Answer from the drawing. Dimensions are ordinates in mm from the lowest x, y and z of the part. Coordinates: 2 decimals unless noted, no trailing zeros. Write each loop counter-clockwise with the first axis right and the second up, starting at its lowest first coordinate (ties: lowest second). Pieces come first, ordered by that corner, then holes. Notation, with made-up numbers: (-25, 89.5) - (22, 89.5) arc R12 ccw to (22, 106.5) - close; hole circle Ø8 at (-14, -26). An arc over 180 degrees is marked (long way). Return JSON: item names as keys, results as strings.
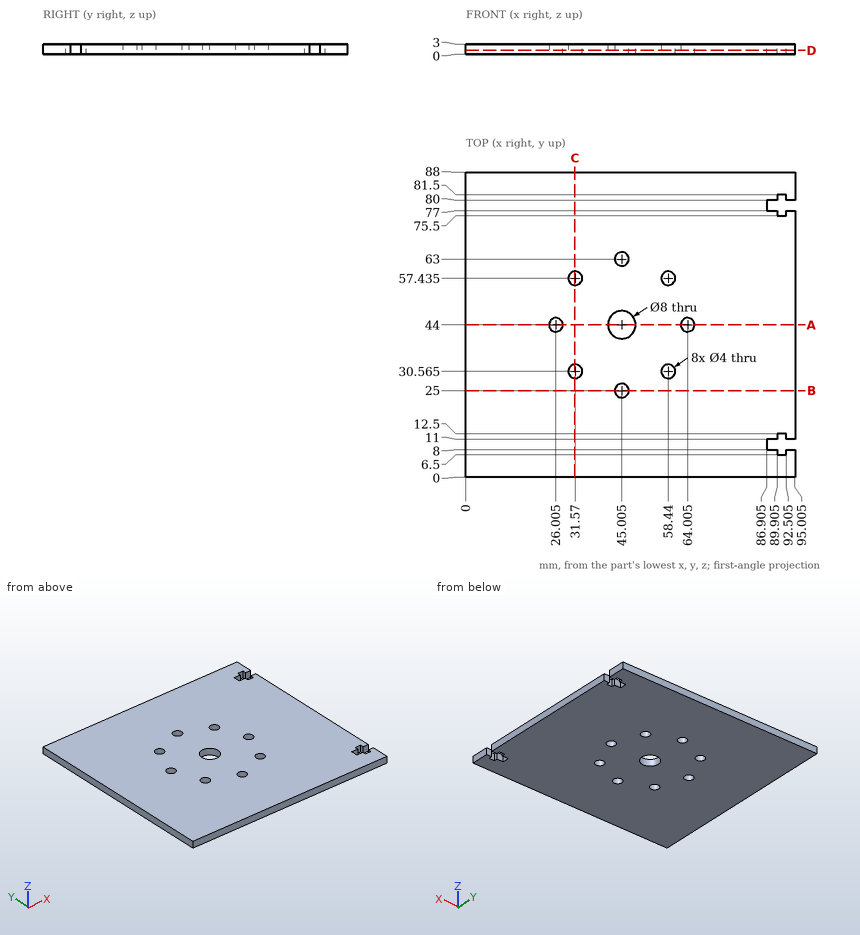
(1) A cutting plane is placed at B-B (y = 25). Determine the outline of the cut face in (x, z) (1 decimal), and give its area (3 significant figures).
Answer:
{"outline": "(0, 0) - (43, 0) - (43, 3) - (0, 3) - close; (47, 0) - (95, 0) - (95, 3) - (47, 3) - close", "area": "273 mm²"}
(2) Flat-ended cylindrical pins translate along their axes: P1, Ø0.9, axis at y = 9.5, z = 1.5, coming from the +X side (1 decimal); P2, Ø0.8, axis at x = 94, z = 2, coming from the -Y side. Find the tip coordinate at first contact, or state that the pin passes through.
Answer:
{"P1": "x = 86.9", "P2": "y = 0"}
(3) A cutting plane is placed at C-C (x = 31.5). Determine the outline of the cut face in (y, z).
Answer:
{"outline": "(0, 0) - (28.57, 0) - (28.57, 3) - (0, 3) - close; (32.56, 0) - (55.44, 0) - (55.44, 3) - (32.56, 3) - close; (59.43, 0) - (88, 0) - (88, 3) - (59.43, 3) - close"}
(4) Straight lines are drawn through the part: line 1 (Y direction, x = 88, z = 1.7); line 2 (X direction, y = 56, z = 2.85) (1 decimal); line 3 (X direction, y = 44.5, z = 2.7) (1 decimal). For each, find the intervals that lie inside material, in ascending order. Write a range as from..to.
Answer:
{"line 1": "0..8, 11..77, 80..88", "line 2": "0..30.2, 33..57, 59.8..95", "line 3": "0..24.1, 27.9..41, 49..62.1, 65.9..95"}
(5) A cutting plane is placed at A-A (y = 44). Determine the outline of the cut face in (x, z) (1 decimal), and give its area (3 significant figures).
Answer:
{"outline": "(0, 0) - (24, 0) - (24, 3) - (0, 3) - close; (28, 0) - (41, 0) - (41, 3) - (28, 3) - close; (49, 0) - (62, 0) - (62, 3) - (49, 3) - close; (66, 0) - (95, 0) - (95, 3) - (66, 3) - close", "area": "237 mm²"}
(6) A cutting plane is placed at D-D (z = 1.15). State how many separate pieces and enclosed holes the cut face has, and give its area (3 significant figures).
Answer:
{"separate pieces": "1", "enclosed holes": "9", "area": "8,150 mm²"}
